```python
from build123d import *

# Parameters (mm, degrees)
SKETCH1_W                             = 1206.5
SKETCH1_H                             = 596.9
BOSS_EXTRUDE1_DEPTH                   = 17.78
F_1_8_0_125_DIAMETER_HOLE1_D          = 3.175
FILLET1_R                             = 6.35
SKETCH4_W                             = 158.75
SKETCH4_H                             = 66.04
SKETCH4_W_2                           = 76.2
SKETCH4_H_2                           = 133.35
CUT_EXTRUDE1_DEPTH                    = 12.7
FILLET2_R                             = 6.35
SKETCH6_W                             = 1.5875
SKETCH6_H                             = 5.08
F_1_8_0_125_DIAMETER_HOLE2_AT_2_COUNT = 2
F_1_8_0_125_DIAMETER_HOLE2_AT_2_PITCH = 1123.95
F_1_8_0_125_DIAMETER_HOLE2_AT_3_COUNT = 2
F_1_8_0_125_DIAMETER_HOLE2_AT_3_PITCH = 1133.602
F_1_8_0_125_DIAMETER_HOLE2_AT_4_COUNT = 2
F_1_8_0_125_DIAMETER_HOLE2_AT_4_PITCH = 1143.254
F_1_8_0_125_DIAMETER_HOLE2_AT_5_COUNT = 2
F_1_8_0_125_DIAMETER_HOLE2_AT_5_PITCH = 618.636019724
F_1_8_0_125_DIAMETER_HOLE2_AT_6_COUNT = 2
F_1_8_0_125_DIAMETER_HOLE2_AT_6_PITCH = 19.05
F_1_8_0_125_DIAMETER_HOLE2_AT_7_COUNT = 2
F_1_8_0_125_DIAMETER_HOLE2_AT_7_PITCH = 9.525


with BuildPart() as part:
    # Sketch1 → Boss-Extrude1 (new body)
    with BuildSketch(Plane(origin=(0, 0, 0), x_dir=(1, 0, 0), z_dir=(0, 1, 0))):
        Rectangle(SKETCH1_W, SKETCH1_H)
    extrude(amount=BOSS_EXTRUDE1_DEPTH)

    # 1/8 (0.125) Diameter Hole1 (through all)
    with Locations(Plane(origin=(0, 17.78, 0), x_dir=(1, 0, 0), z_dir=(0, 1, 0))):
        with Locations((0, 0), (457.2, 152.4), (-457.2, -152.4), (-457.2, 152.4), (457.2, -152.4)):
            Hole(F_1_8_0_125_DIAMETER_HOLE1_D / 2)

    # Fillet1
    fillet1_edges = [part.edges().sort_by_distance(p)[0] for p in [
        (603.25, 8.89, 298.45),
        (-603.25, 8.89, 298.45),
        (-603.25, 8.89, -298.45),
        (603.25, 8.89, -298.45),
    ]]
    fillet(fillet1_edges, radius=FILLET1_R)

    # Sketch4 → Cut-Extrude1 (cut)
    with BuildSketch(Plane(origin=(0, 17.78, 0), x_dir=(1, 0, 0), z_dir=(0, 1, 0))):
        with Locations((0, -265.43)):
            Rectangle(SKETCH4_W, SKETCH4_H)
        with Locations((-565.15, 0)):
            Rectangle(SKETCH4_W_2, SKETCH4_H_2)
    extrude(amount=-CUT_EXTRUDE1_DEPTH, mode=Mode.SUBTRACT)

    # Fillet2
    fillet2_edges = [part.edges().sort_by_distance(p)[0] for p in [
        (79.375, 11.43, 232.41),
        (79.375, 11.43, 298.45),
        (-79.375, 11.43, 298.45),
        (-79.375, 11.43, 232.41),
        (-603.25, 11.43, 66.675),
        (-603.25, 11.43, -66.675),
        (-527.05, 11.43, -66.675),
        (-527.05, 11.43, 66.675),
    ]]
    fillet(fillet2_edges, radius=FILLET2_R)

    # Sketch6 → 1/8 (0.125) Diameter Hole2 (revolve, cut)
    with BuildSketch(Plane(origin=(558.8, 5.08, 0), x_dir=(0, 0, 1), z_dir=(1, 0, 0))):
        with Locations((0.79375, 2.54)):
            Rectangle(SKETCH6_W, SKETCH6_H)
    f_1_8_0_125_diameter_hole2 = revolve(axis=Axis((558.8, 11.43, 0), (0, -1, 0)), mode=Mode.SUBTRACT)

    # 1/8 (0.125) Diameter Hole2 at 2: 1/8 (0.125) Diameter Hole2 ×2
    with Locations(*[(-i * F_1_8_0_125_DIAMETER_HOLE2_AT_2_PITCH, 0, 0) for i in range(1, F_1_8_0_125_DIAMETER_HOLE2_AT_2_COUNT)]):
        add(f_1_8_0_125_diameter_hole2, mode=Mode.SUBTRACT)

    # 1/8 (0.125) Diameter Hole2 at 3: 1/8 (0.125) Diameter Hole2 ×2
    with Locations(*[(-i * F_1_8_0_125_DIAMETER_HOLE2_AT_3_PITCH, 0, 0) for i in range(1, F_1_8_0_125_DIAMETER_HOLE2_AT_3_COUNT)]):
        add(f_1_8_0_125_diameter_hole2, mode=Mode.SUBTRACT)

    # 1/8 (0.125) Diameter Hole2 at 4: 1/8 (0.125) Diameter Hole2 ×2
    with Locations(*[(-i * F_1_8_0_125_DIAMETER_HOLE2_AT_4_PITCH, 0, 0) for i in range(1, F_1_8_0_125_DIAMETER_HOLE2_AT_4_COUNT)]):
        add(f_1_8_0_125_diameter_hole2, mode=Mode.SUBTRACT)

    # 1/8 (0.125) Diameter Hole2 at 5: 1/8 (0.125) Diameter Hole2 ×2
    with Locations(*[Vector(-0.9032775043542898, 0, 0.4290568145682877) * (i * F_1_8_0_125_DIAMETER_HOLE2_AT_5_PITCH) for i in range(1, F_1_8_0_125_DIAMETER_HOLE2_AT_5_COUNT)]):
        add(f_1_8_0_125_diameter_hole2, mode=Mode.SUBTRACT)

    # 1/8 (0.125) Diameter Hole2 at 6: 1/8 (0.125) Diameter Hole2 ×2
    with Locations(*[(i * F_1_8_0_125_DIAMETER_HOLE2_AT_6_PITCH, 0, 0) for i in range(1, F_1_8_0_125_DIAMETER_HOLE2_AT_6_COUNT)]):
        add(f_1_8_0_125_diameter_hole2, mode=Mode.SUBTRACT)

    # 1/8 (0.125) Diameter Hole2 at 7: 1/8 (0.125) Diameter Hole2 ×2
    with Locations(*[(i * F_1_8_0_125_DIAMETER_HOLE2_AT_7_PITCH, 0, 0) for i in range(1, F_1_8_0_125_DIAMETER_HOLE2_AT_7_COUNT)]):
        add(f_1_8_0_125_diameter_hole2, mode=Mode.SUBTRACT)


solid = part.part
```
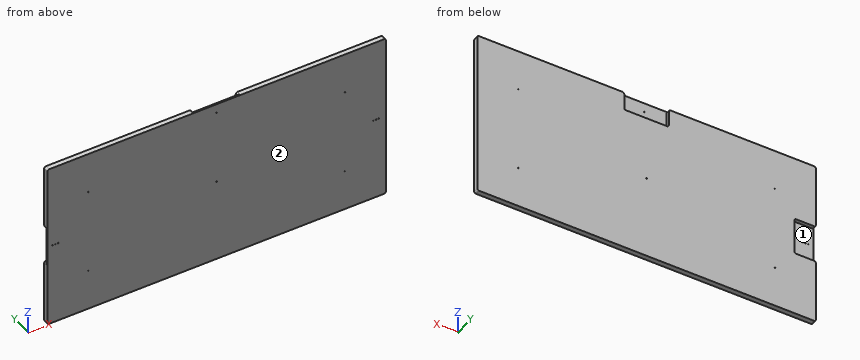
Can you work these out from the model? Positions are in its coordinate system, mm. Face numbers are marked on the shaded views. Round coordinates to 2 decimals unless told otherwise and drop trailing zeros. Loops run counter-clockwise (first coordinate to the right, second up) from the corner with the lowest first, then second, coordinate; pieces in that order, holes last. Notation, with made-up numbers: M -28.75,89.25 L -24.75,89.25 A7 cw -24.75,98.25 Z; hole C 3,26.25 d3. An arc over 180 degrees is marked long. Write item = value, one per line. Start each with the question number.
(1) Suppose I cut it at A-A on y = 8.75. Give the number of separate pieces and of enclosed holes in the cut face, plus the area to 3 significant figures.
(2) If we mould it in two halves opening along Z, with no side actions, what happens to the marked faces 1 and 2? For each: released by +Z, released by -Z, zero draft, split by the parting line, or undercut.
(3) I'm going to push flat-ended pins straight in: P1, Ø3, axis at x = -346.5, z = 46, coming from the -Y side; P2, Ø1, axis at x = 568, z = -0.5, coming from the -Y side; P3, Ø1.5, axis at x = 12, y = 8, coming from the +Z side; P4, Ø2.5, axis at x = 0, z = 265.43, coming from the +Y side. Where does each tip first touch, or does it pass through?
(4) I need wall thicknesses on line 1 along Z through (x, y) = (-457.2, 8); line 2 along X through (y, z) = (8, 152.4); line 3 along Z through (x, y) = (-550.5, 15.25) (3 decimals). Which ranges of each line are inside material? Lowest first, please.
(5) Suppose I cut it at B-B on x = -32. Write out the boundary of the cut face in (y, z).
Answer block:
q1.separate_pieces = 1
q1.enclosed_holes = 5
q1.area = 699,000 mm²
q2.face_1 = undercut
q2.face_2 = zero draft
q3.P1 = 0
q3.P2 = 5.08
q3.P3 = 232.41
q3.P4 = through
q4.line_1 = -298.45 to -153.99, -150.81 to 150.81, 153.99 to 298.45
q4.line_2 = -603.25 to -458.79, -455.61 to 455.61, 458.79 to 603.25
q4.line_3 = -298.45 to -66.675, 66.675 to 298.45
q5.outline = M 0,-298.45 L 17.78,-298.45 L 17.78,232.41 L 5.08,232.41 L 5.08,298.45 L 0,298.45 Z
